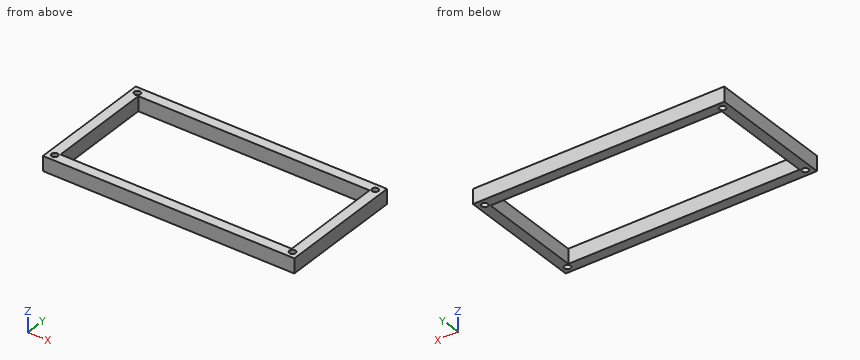
Autodesk Inventor part; units mm, degrees
ref_plane "YZ Plane" through (0, 0, 0) normal (1, 0, 0) x (0, 1, 0)
ref_plane "XZ Plane" through (0, 0, 0) normal (0, 1, 0) x (-1, 0, 0)
ref_plane "XY Plane" through (0, 0, 0) normal (0, 0, 1) x (1, 0, 0)
sketch "Sketch1" plane through (0, 0, 0) normal (0, 0, 1) x (1, 0, 0)
  line L0 (-25.2, 25.2) -> (25.2, 25.2)
  line L1 (25.2, 25.2) -> (25.2, -25.2)
  line L2 (25.2, -25.2) -> (-25.2, -25.2)
  line L3 (-25.2, -25.2) -> (-25.2, 25.2)
  line L4 (-25.2, 25.2) -> (25.2, -25.2) construction
  line L5 (25.2, 25.2) -> (-25.2, -25.2) construction
  line L6 (-30, 30) -> (30, 30)
  line L7 (30, 30) -> (30, -30)
  line L8 (30, -30) -> (-30, -30)
  line L9 (-30, -30) -> (-30, 30)
  line L10 (-30, 30) -> (30, -30) construction
  line L11 (30, 30) -> (-30, -30) construction
  line L12 (-30, 30) -> (-26.768, 30)
  line L13 (-26.768, 30) -> (-26.768, 26.768)
  circle A0 centre (-26.768, 26.768) radius 1.5
  circle A1 centre (-26.768, -26.768) radius 1.5
  circle A2 centre (26.768, -26.768) radius 1.5
  circle A3 centre (26.768, 26.768) radius 1.5
  line L14 (85.2, 25.2) -> (34.8, 25.2)
  line L15 (34.8, 25.2) -> (34.8, -25.2)
  line L16 (34.8, -25.2) -> (85.2, -25.2)
  line L17 (85.2, -25.2) -> (85.2, 25.2)
  line L18 (85.2, 25.2) -> (34.8, -25.2) construction
  line L19 (34.8, 25.2) -> (85.2, -25.2) construction
  line L20 (90, 30) -> (30, 30)
  line L21 (30, -30) -> (90, -30)
  line L22 (90, -30) -> (90, 30)
  line L23 (90, 30) -> (30, -30) construction
  line L24 (30, 30) -> (90, -30) construction
  line L25 (90, 30) -> (86.768, 30)
  line L26 (86.768, 30) -> (86.768, 26.768)
  circle A4 centre (86.768, 26.768) radius 1.5
  circle A5 centre (86.768, -26.768) radius 1.5
  line L27 (25.2, 25.2) -> (34.8, 25.2)
  line L28 (25.2, -25.2) -> (34.8, -25.2)
  point P0 (0, 0)
  point P1 (60, 0)
  dimension "d0" = 50.4
  dimension "d1" = 50.4
  dimension "d2" = 60
  dimension "d3" = 60
  dimension "d4" = 3.232
  dimension "d5" = 3.232
  dimension "d6" = 3
  dimension "d9" = 360
extrude "Extrusion1" add sketch "Sketch1" along normal blind 7 contours L3 L2 L28 L7 L8 L9 L6 L27 L0 | L7 L20 L22 L21 L28 L16 L17 L14 L27 | A2 | A3
properties part number "rack_C2x1"
Work out the finished part from the listing and answer in its coordinate system (mm). Round coordinates to 2 decimals unless told otherwise and drop trailing zeros. Loops run counter-clockwise (first coordinate to the right, second up) from the corner with the lowest first, then second, coordinate; pieces in that order, holes last. Notation, with made-up numbers: (17, 4.5) - (76, 4.5) arc R26 cw to (76, 35.5) - close; hole circle Ø5 at (27, -13.5). An arc over 180 degrees is marked (long way). Use one line per item in the form item = value. Start each with the question number.
(1) Consider line 1 (X direction, y = -16, z = 6.5); line 2 (Y direction, x = -20.5, z = 5.5). Determine where each line is inside the solid, lowest interval first.
(2) Find section B-B on x = -9. Determine the outline of the cut face in (y, z), and give its area (3 significant figures).
(3) Find section A-A on y = -23.5. Determine the outline of the cut face in (x, z).
(4) Find section C-C on z = 5. Determine the outline of the cut face in (x, y).
Answer list:
q1.line_1 = -30 to -25.2, 85.2 to 90
q1.line_2 = -30 to -25.2, 25.2 to 30
q2.outline = (-30, 0) - (-25.2, 0) - (-25.2, 7) - (-30, 7) - close; (25.2, 0) - (30, 0) - (30, 7) - (25.2, 7) - close
q2.area = 67.2 mm^2
q3.outline = (-30, 0) - (-25.2, 0) - (-25.2, 7) - (-30, 7) - close; (85.2, 0) - (90, 0) - (90, 7) - (85.2, 7) - close
q4.outline = (-30, -30) - (90, -30) - (90, 30) - (-30, 30) - close; hole circle Ø3 at (-26.77, -26.77); hole circle Ø3 at (-26.77, 26.77); hole (-25.2, -25.2) - (85.2, -25.2) - (85.2, 25.2) - (-25.2, 25.2) - close; hole circle Ø3 at (86.77, -26.77); hole circle Ø3 at (86.77, 26.77)
